from build123d import *

# Parameters (mm, degrees)
ESQUISSE1_W             = 660
ESQUISSE1_H             = 1010
BOSS_EXTRU_1_DEPTH      = 10
ENL_V_MAT_EXTRU_1_DEPTH = 5
CHANFREIN1_SIZE         = 5


with BuildPart() as part:
    # Esquisse1 → Boss.-Extru.1 (new body)
    with BuildSketch(Plane.XY):
        with Locations((330, 505)):
            Rectangle(ESQUISSE1_W, ESQUISSE1_H)
    extrude(amount=BOSS_EXTRU_1_DEPTH)

    # Esquisse2 → Enlèv. mat.-Extru.1 (cut)
    with BuildSketch(Plane.XY.offset(10)):
        Polygon((120, 328.492424049), (120, 681.507575951), (60, 741.507575951), (60, 268.492424049), align=None)
        Polygon((268.492424049, 830), (391.507575951, 830), (511.507575951, 950), (148.492424049, 950), align=None)
        Polygon((60, 950), (60, 783.933982822), (150, 693.933982822), (150, 316.066017178), (60, 226.066017178), (60, 60), (106.066017178, 60), (256.066017178, 210), (403.933982822, 210), (553.933982822, 60), (600, 60), (600, 226.066017178), (510, 316.066017178), (510, 693.933982822), (600, 783.933982822), (600, 950), (553.933982822, 950), (403.933982822, 800), (256.066017178, 800), (106.066017178, 950), align=None)
        Polygon((540, 328.492424049), (540, 681.507575951), (600, 741.507575951), (600, 268.492424049), align=None)
        Polygon((511.507575951, 60), (148.492424049, 60), (268.492424049, 180), (391.507575951, 180), align=None)
    extrude(amount=-ENL_V_MAT_EXTRU_1_DEPTH, mode=Mode.SUBTRACT)

    # Chanfrein1
    chanfrein1_edges = [part.edges().sort_by_distance(p)[0] for p in [
        (330, 60, 5),
        (208.492424049, 120, 5),
        (330, 180, 5),
        (451.507575951, 120, 5),
        (60, 505, 5),
        (90, 711.507575951, 5),
        (120, 505, 5),
        (90, 298.492424049, 5),
        (600, 505, 5),
        (570, 298.492424049, 5),
        (540, 505, 5),
        (570, 711.507575951, 5),
        (181.066017178, 875, 5),
        (330, 800, 5),
        (478.933982822, 875, 5),
        (576.966991411, 950, 5),
        (600, 866.966991411, 5),
        (555, 738.933982822, 5),
        (510, 505, 5),
        (555, 271.066017178, 5),
        (600, 143.033008589, 5),
        (576.966991411, 60, 5),
        (478.933982822, 135, 5),
        (330, 210, 5),
        (181.066017178, 135, 5),
        (83.033008589, 60, 5),
        (60, 143.033008589, 5),
        (105, 271.066017178, 5),
        (150, 505, 5),
        (105, 738.933982822, 5),
        (60, 866.966991411, 5),
        (83.033008589, 950, 5),
        (330, 950, 5),
        (451.507575951, 890, 5),
        (330, 830, 5),
        (208.492424049, 890, 5),
    ]]
    chamfer(chanfrein1_edges, length=CHANFREIN1_SIZE - 0.0001)  # a hair under: the kernel refuses the full size


solid = part.part
Could you check a few things on this model? Use its own coordinates, in mm. Give positions to 0.01 mm unless a question says otherwise; leave off trailing zeros.
Item 1: If we mould it in two halves opening along X, with no side actions, what happens to faces 1 (the face through (87.788, 299.865, 7.465)), 2 (the face through (105, 737, 10)), 3 (the face through (181.066, 871.415, 7.465))? For each: pulls with the +X half, pulls with the -X half, needs draft (parallel to the pull), parting line crosses it, or undercut.
Item 2: I need wall thicknesses on line 1 (X direction, y = 912, z = 9.5); line 2 (X direction, y = 479, z = 7); line 3 (Y direction, x = 225, z = 8.25). Which ranges of each line are inside material? Lowest first, please.
Item 3: I'm going to push flat-ended pins straight in: pin 1 (1.5 mm diameter, centred on x = 174, y = 320, fed in from +Z); pin 2 (2 mm diameter, centred on y = 406, z = 7.5, fed in from -X). Where does each tip first touch, or does it pass through?
Item 4: If we section it at C-C, the plane z = 8: Count the separate pieces of the cut face and the enclosed holes in it, plus the area to 3 significant figures.
Values:
1. face 1: undercut
1. face 2: needs draft
1. face 3: undercut
2. line 1: x = 0 to 60.5, 143.36 to 187.2, 472.8 to 516.64, 599.5 to 660
2. line 2: x = 0 to 63, 117 to 153, 507 to 543, 597 to 660
2. line 3: y = 0 to 61.75, 134.03 to 181.41, 828.59 to 875.97, 948.25 to 1010
3. pin 1: stops at z = 5
3. pin 2: stops at x = 0
4. separate pieces: 1
4. enclosed holes: 5
4. area: 265,000 mm2
